```python
from build123d import *

# Parameters (mm, degrees)
F0_R     = 1.875
F1_DEPTH = 10
F0_R_2   = 3.75
F2_DEPTH = 1
F4_DEPTH = 2


with BuildPart() as f1:
    # F0 (on Top) → F1 (new body)
    with BuildSketch(Plane.XY):
        Circle(F0_R)
    extrude(amount=F1_DEPTH)

    # F0 (on Top) → F2 (join)
    with BuildSketch(Plane.XY):
        Circle(F0_R_2)
        Circle(F0_R, mode=Mode.SUBTRACT)
    extrude(amount=F2_DEPTH)

    # F3 (on face) → F4 (cut)
    with BuildSketch(Plane.XY.offset(10)):
        with BuildLine():
            Line((-0.25, 1.8582585934), (-0.25, -1.8582585934))
            ThreePointArc((-0.25, -1.8582585934), (0, -1.875), (0.25, -1.8582585934))
            Line((0.25, -1.8582585934), (0.25, 1.8582585934))
            ThreePointArc((0.25, 1.8582585934), (0, 1.875), (-0.25, 1.8582585934))
        make_face()
        with BuildLine():
            Line((-0.25, 2.5), (-0.25, 1.8582585934))
            ThreePointArc((-0.25, 1.8582585934), (0, 1.875), (0.25, 1.8582585934))
            Line((0.25, 1.8582585934), (0.25, 2.5))
            Line((0.25, 2.5), (-0.25, 2.5))
        make_face()
    extrude(amount=-F4_DEPTH, mode=Mode.SUBTRACT)


solid = f1.part
```
The model under review builds one solid part; all positions refer to its coordinate system, in mm. A direction names the side the tool comes from. Coordinates: 2 decimals unless noted, no trailing zeros. Write each loop counter-clockwise with the first axis right and the second up, starting at its lowest first coordinate (ties: lowest second). Pieces come first, ordered by that corner, then holes.
1) Clearance check with flat-ended pins moving along their axes: pin 1 Ø3 at (x, y) = (-1, 0.5) entering from -Z; pin 2 Ø2 at (y, z) = (-0.5, 8.5) entering from -X (3 decimals); pin 3 Ø2 at (y, z) = (2, 8.5) entering from +X; pin 4 Ø1.6 at (y, z) = (-1, 9.5) entering from +X. State where each tip first meets the part, or that it passes through.
2) Machinability: for faces 1 (the face through (1, 0, 10)), 2 (the face through (-0.41, -1.83, 5.44)), 3 (the face through (-0.25, 0, 9)), which of the approach directions +Z, -Z, +X, -X, +Y, -Y give a long, thin tool a straight path to every point of the face, cutting with its end or side? Answer none if there is none.
3) We need section B-B on z = 9.25. State the section outline as (x, y) points (3 decimals), then the cut area to 3 significant figures.
4) To check wall thickness, follow probe 1 along Z at (x, y) = (2.75, 0.5); probe 2 along X at (y, z) = (-0.75, 9); probe 3 along Z at (x, y) = (0, -1.75). State the ranges of each line that lie inside material, in increasing order.
5) We need section D-D on z = 4.25. State the section outline as (x, y) points (3 decimals), then the cut area to 3 significant figures.
6) We need section C-C on x = 0. State the section outline as (y, z) points (3 decimals), then the cut area to 4 significant figures.
7) We need section A-A on y = 0. State the section outline as (x, z) points (3 decimals).
8) The part is to be moulded in two halves that separate along X. For faces 4 (the face through (1, 2, 1)), 5 (the face through (0.25, 0, 9)), 6 (the face through (-3.746, 0.165, 0.493)), say which applies: pulls with the +X half, pulls with the -X half, needs draft (parallel to the pull), parting line crosses it, or undercut.
Answer list:
1. pin 1: stops at z = 0
1. pin 2: stops at x = -1.875
1. pin 3: stops at x = 1.59
1. pin 4: stops at x = 1.86
2. face 1: +Z, +X, -X, +Y, -Y
2. face 2: +Z
2. face 3: +Z, +Y, -Y
3. outline: (-0.25, -1.858) - (-0.25, 1.858) arc R1.875 ccw to start; (0.25, -1.858) arc R1.875 ccw to (0.25, 1.858) - close
3. area: 9.18 mm2
4. probe 1: z = 0 to 1
4. probe 2: x = -1.72 to -0.25, 0.25 to 1.72
4. probe 3: z = 0 to 8
5. outline: circle Ø3.75 at (0, 0)
5. area: 11.0 mm2
6. outline: (-3.75, 0) - (3.75, 0) - (3.75, 1) - (1.875, 1) - (1.875, 8) - (-1.875, 8) - (-1.875, 1) - (-3.75, 1) - close
6. area: 33.75 mm2
7. outline: (-3.75, 0) - (3.75, 0) - (3.75, 1) - (1.875, 1) - (1.875, 10) - (0.25, 10) - (0.25, 8) - (-0.25, 8) - (-0.25, 10) - (-1.875, 10) - (-1.875, 1) - (-3.75, 1) - close
8. face 4: needs draft
8. face 5: undercut
8. face 6: parting line crosses it
